Design review of the part built by this model. Coordinates are the model's own, in mm. A direction names the side the tool comes from. Coordinates: 2 decimals unless noted, no trailing zeros. Write each loop counter-clockwise with the first axis right and the second up, starting at its lowest first coordinate (ties: lowest second). Pieces come first, ordered by that corner, then holes. Notation, with made-up numbers: (-17, 18.5) -> (15, 18.5) arc R26 ccw to (15, 38.5) -> close; hole circle Ø5 at (71, -13). An arc over 180 degrees is marked (long way). Return JSON: item names as keys, results as strings. Group by question number.
from build123d import *

# Parameters (mm, degrees)
SKETCH_1_R          = 4.025
EXTRUDE_1_DEPTH     = 4
CUT_EXTRUDE_START   = -10
CUT_EXTRUDE_1_DEPTH = 10
SKETCH_4_R          = 5.05
CUT_EXTRUDE_2_DEPTH = 1
CUT_EXTRUDE_START_2 = -2
CUT_EXTRUDE_3_DEPTH = 2
FILLET_2_R          = 2


with BuildPart() as part:
    # 草图1 → 凸台-拉伸1 (new body)
    with BuildSketch(Plane.XY):
        with BuildLine():
            Line((-30, 7.5), (30, 7.5))
            ThreePointArc((30, 7.5), (37.5, 0), (30, -7.5))
            Line((30, -7.5), (-30, -7.5))
            ThreePointArc((-30, -7.5), (-37.5, 0), (-30, 7.5))
        make_face()
        with Locations((-30, 0)):
            Circle(SKETCH_1_R, mode=Mode.SUBTRACT)
        with Locations((30, 0)):
            Circle(SKETCH_1_R, mode=Mode.SUBTRACT)
    extrude(amount=EXTRUDE_1_DEPTH)

    # 草图2 → 切除-拉伸1 (cut)
    with BuildSketch(Plane.XY.offset(4).offset(CUT_EXTRUDE_START)):
        with BuildLine():
            ThreePointArc((-26.39526938, 6.576923077), (-20.581237378, 4.281443859), (-14.379500648, 3.5))
            Line((-14.379500648, 3.5), (14.379500648, 3.5))
            ThreePointArc((14.379500648, 3.5), (20.581237378, 4.281443859), (26.39526938, 6.576923077))
            ThreePointArc((26.39526938, 6.576923077), (28.139478981, 7.265566842), (30, 7.5))
            Line((30, 7.5), (-30, 7.5))
            ThreePointArc((-30, 7.5), (-28.139478981, 7.265566842), (-26.39526938, 6.576923077))
        make_face()
        with BuildLine():
            ThreePointArc((-26.39526938, -6.576923077), (-28.139478981, -7.265566842), (-30, -7.5))
            Line((-30, -7.5), (30, -7.5))
            ThreePointArc((30, -7.5), (28.139478981, -7.265566842), (26.39526938, -6.576923077))
            ThreePointArc((26.39526938, -6.576923077), (20.581237378, -4.281443859), (14.379500648, -3.5))
            Line((14.379500648, -3.5), (-14.379500648, -3.5))
            ThreePointArc((-14.379500648, -3.5), (-20.581237378, -4.281443859), (-26.39526938, -6.576923077))
        make_face()
    extrude(amount=CUT_EXTRUDE_1_DEPTH, mode=Mode.SUBTRACT)

    # 草图4 → 切除-拉伸2 (cut)
    with BuildSketch(Plane(origin=(0, 0, 0), x_dir=(-1, 0, 0), z_dir=(0, 0, -1))):
        with Locations((30, 0)):
            Circle(SKETCH_4_R)
    extrude(amount=-CUT_EXTRUDE_2_DEPTH, mode=Mode.SUBTRACT)

    # 草图5 → 切除-拉伸3 (cut)
    with BuildSketch(Plane.XY.offset(4).offset(CUT_EXTRUDE_START_2)):
        with BuildLine():
            ThreePointArc((-23.103831173, -2.948364888), (-18.801369709, -1.864552303), (-14.379500648, -1.5))
            Line((-14.379500648, -1.5), (14.379500648, -1.5))
            ThreePointArc((14.379500648, -1.5), (18.801369709, -1.864552303), (23.103831173, -2.948364888))
            ThreePointArc((23.103831173, -2.948364888), (22.5, 0), (23.103831173, 2.948364888))
            ThreePointArc((23.103831173, 2.948364888), (18.801369709, 1.864552303), (14.379500648, 1.5))
            Line((14.379500648, 1.5), (-14.379500648, 1.5))
            ThreePointArc((-14.379500648, 1.5), (-18.801369709, 1.864552303), (-23.103831173, 2.948364888))
            ThreePointArc((-23.103831173, 2.948364888), (-22.65250838, 1.504781346), (-22.5, 0))
            ThreePointArc((-22.5, 0), (-22.65250838, -1.504781346), (-23.103831173, -2.948364888))
        make_face()
    extrude(amount=CUT_EXTRUDE_3_DEPTH, mode=Mode.SUBTRACT)

    # 圆角2
    fillet_2_edges = [part.edges().sort_by_distance(p)[0] for p in [
        (23.103831173, 2.948364888, 3),
        (23.103831173, -2.948364888, 3),
        (-23.103831173, -2.948364888, 3),
        (-23.103831173, 2.948364888, 3),
    ]]
    fillet(fillet_2_edges, radius=FILLET_2_R)


solid = part.part
Q1. For P1, Ø2, axis at x = 6.5, z = 2, coming from the -Y side; P2, Ø0.6, axis at x = -2.5, z = 3, coming from the +Y side; P3, Ø2, axis at y = 5.5, z = 0.5, coming from the -X side; P4, Ø1, axis at x = 27, y = 1, coming from the +Z side, all flat-tipped, find the tip position at first contact; note any pin that passes through.
Q2. The part is to be moulded in two halves that separate along X. For faces 1 (the flat face through (1, 2, 4)), 2 (the cylindrical face through (20.666, -4.303, 1.972)), say which applies: +X half, -X half, draft (parallel to the pull), parting line (faces both ways), or undercut.
Q3. We need section B-B on x = 19. Write out the cut boundary in (y, z), plus the area to 3 significant figures.
Q4. We need section A-A on x = 0. Write out the cut boundary in (y, z), plus the area to 3 significant figures.
Q5. Wall thickness on L1, parallel to Y at x = -30, z = 1.75 (3 decimals); L2, parallel to Y at x = -30, z = 0.7; L3, parallel to X at y = -0.5, z = 3.4: over which ranges is each line inside the solid? List them lowest first.
Q6. For faces 3 (the cylindrical face through (-20.5, -4.26, 1.97)), 4 (the cylindrical face through (20.5, 4.26, 1.97)), 5 (the cylindrical face through (-17.21, 1.65, 2.99)), list the 3-axis set-ups (+Z, -Z, +X, -X, +Y, -Y) from which the entire face can be reached by the end or side of a thin tool; tool diameter is ignored.
Findings below:
{
 "1": {"P1": "stops at y = -3.5", "P2": "stops at y = 3.5", "P3": "stops at x = -36", "P4": "passes through"},
 "2": {"face 1": "draft", "face 2": "undercut"},
 "3": {"outline": "(-3.93, 0) -> (3.93, 0) -> (3.93, 4) -> (1.9, 4) -> (1.9, 2) -> (-1.9, 2) -> (-1.9, 4) -> (-3.93, 4) -> close", "area": "23.9 mm^2"},
 "4": {"outline": "(-3.5, 0) -> (3.5, 0) -> (3.5, 4) -> (1.5, 4) -> (1.5, 2) -> (-1.5, 2) -> (-1.5, 4) -> (-3.5, 4) -> close", "area": "22.0 mm^2"},
 "5": {"L1": "y = -7.5 to -4.025, 4.025 to 7.5", "L2": "y = -7.5 to -5.05, 5.05 to 7.5", "L3": "x = -37.48 to -33.99, -26.01 to -22.47, 22.47 to 26.01, 33.99 to 37.48"},
 "6": {"face 3": "+Z, -Z, -Y", "face 4": "+Z, -Z, +Y", "face 5": "+Z"}
}
